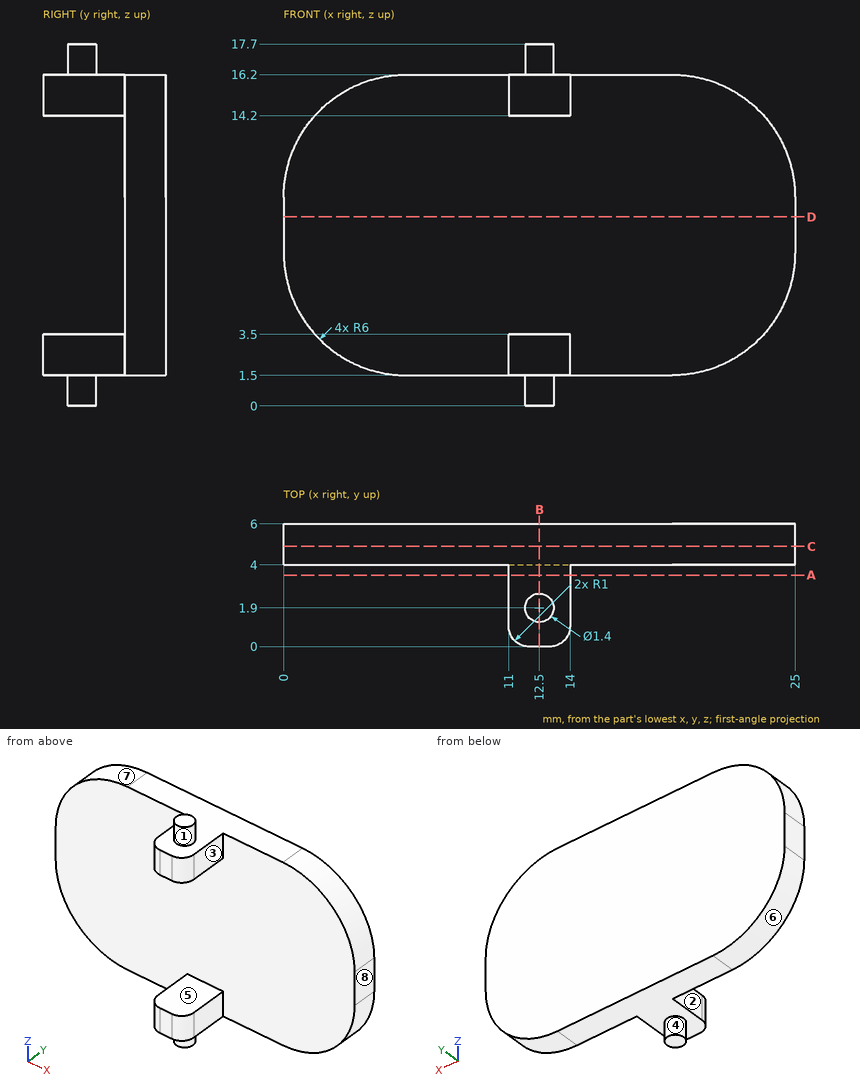
Answer from the drawing. Dimensions are ordinates in mm from the lowest x, y and z of the part. A direction names the side the tool comes from. Round coordinates to 2 decimals unless told otherwise and drop trailing zeros. Loops run counter-clockwise (first coordinate to the right, second up) from the corner with the lowest first, then second, coordinate; pieces in that order, holes last. Notation, with made-up numbers: M 64,42 L 97,42 A24 cw 97,70 Z; hole C -14.75,2 d6. An arc over 180 degrees is marked long. One line per question, with ' | ' between items. Start each with the question number.
(1) A cutting plane is placed at D-D on z = 9.25. Write down the section's boundary in (x, y), plus the area to 3 significant figures.
(2) A cutting plane is placed at C-C on y = 4.9. Write down the section's boundary in (x, z), plus the area to 3 significant figures.
(3) A tool of negligible diameter and unlimited length cuts with its end or side. For the marked faces 1, 2, 3 and 4, from which of +Z, -Z, +X, -X, +Y, -Y can it reach the whole face along a straight path? Write none if from no direction.
(4) Flat-ended cylindrical pins translate along their axes: pin 1 Ø0.6 at (y, z) = (3, 3) entering from -X; pin 2 Ø1.5 at (y, z) = (5, 2.5) entering from +X; pin 3 Ø7.5 at (x, z) = (15, 9.5) entering from -Y. Find the tip coordinate at first contact, or state that the pin passes through.
(5) For a pull along Z with two mould halves and no side action, classify the marked faces 5, 6, 7 and 8 as released by +Z, released by -Z, zero draft, split by the parting line, or undercut.
(6) A cutting plane is placed at B-B on x = 12.5. Write down the section's boundary in (y, z).
(7) Find the intervals of material crossed by line 1 (Y direction, x = 16, z = 14.5); line 2 (Z direction, x = 10, y = 5.45); line 3 (X direction, y = 3.15, z = 14.75), in increasing order.
(8) A cutting plane is placed at A-A on y = 3.5. Write down the section's boundary in (x, z), plus the area to 3 significant figures.
Geometry check:
1) outline: M 0,4 L 25,4 L 25,6 L 0,6 Z | area: 50.0 mm²
2) outline: M 0,7.5 A6 ccw 6,1.5 L 19,1.5 A6 ccw 25,7.5 L 25,10.2 A6 ccw 19,16.2 L 6,16.2 A6 ccw 0,10.2 Z | area: 337 mm²
3) face 1: +Z | face 2: +Z, -Z, -X, -Y | face 3: +Z, -Z, +X, -Y | face 4: -Z
4) pin 1: stops at x = 11 | pin 2: stops at x = 23.24 | pin 3: stops at y = 4
5) face 5: undercut | face 6: released by -Z | face 7: released by +Z | face 8: zero draft
6) outline: M 0,1.5 L 1.2,1.5 L 1.2,0 L 2.6,0 L 2.6,1.5 L 6,1.5 L 6,16.2 L 2.6,16.2 L 2.6,17.7 L 1.2,17.7 L 1.2,16.2 L 0,16.2 L 0,14.2 L 4,14.2 L 4,3.5 L 0,3.5 Z
7) line 1: y = 4 to 6 | line 2: z = 1.5 to 16.2 | line 3: x = 11 to 14
8) outline: M 11,1.5 L 14,1.5 L 14,3.5 L 11,3.5 Z; M 11,14.2 L 14,14.2 L 14,16.2 L 11,16.2 Z | area: 12.0 mm²
